Design review of the part shown in the three views and the two pictorial views. Dimensions are in mm from the part's minimum x, y and z. Round coordinates to 2 decimals unless told otherwise and drop trailing zeros. Loops run counter-clockwise (first coordinate to the right, second up) from the corner with the lowest first, then second, coordinate; pieces in that order, holes last. Notation, with made-up numbers: M -2,82 L 24,82 A7 cw 24,88 Z; hole C 18,86 d5. An arc over 180 degrees is marked long. One line per question, with ' | ' between items. Start each with the question number.
1) We need section C-C (z = 1.95). Give the boundary of the cut face in (x, y) (3 decimals).
2) We need section B-B (x = 50.8). Give the boundary of the cut face in (y, z) (3 decimals), and give its area (3 significant figures).
3) We need section D-D (y = 38.5). Give the boundary of the cut face in (x, z) (3 decimals), and give its area (3 significant figures).
4) For pin 1 Ø4 at (x, y) = (63.5, 38.1) entering from +Z; pin 2 Ø12 at (x, y) = (66.5, 6.5) entering from -Z, all flat-tipped, find the tip position at first contact; note any pin that passes through.
5) For probe 1 along X at (y, z) = (38.1, 2.15) (3 decimals); probe 2 along Y at (x, z) = (50.8, 0.9) (3 decimals); probe 3 along Y at (x, z) = (12.7, 1.2) (3 decimals), list the stretches that pass through material, from the lowest coordinate up. Write a range as from..to.
6) We need section A-A (y = 12.7). Give the boundary of the cut face in (x, z) (3 decimals).
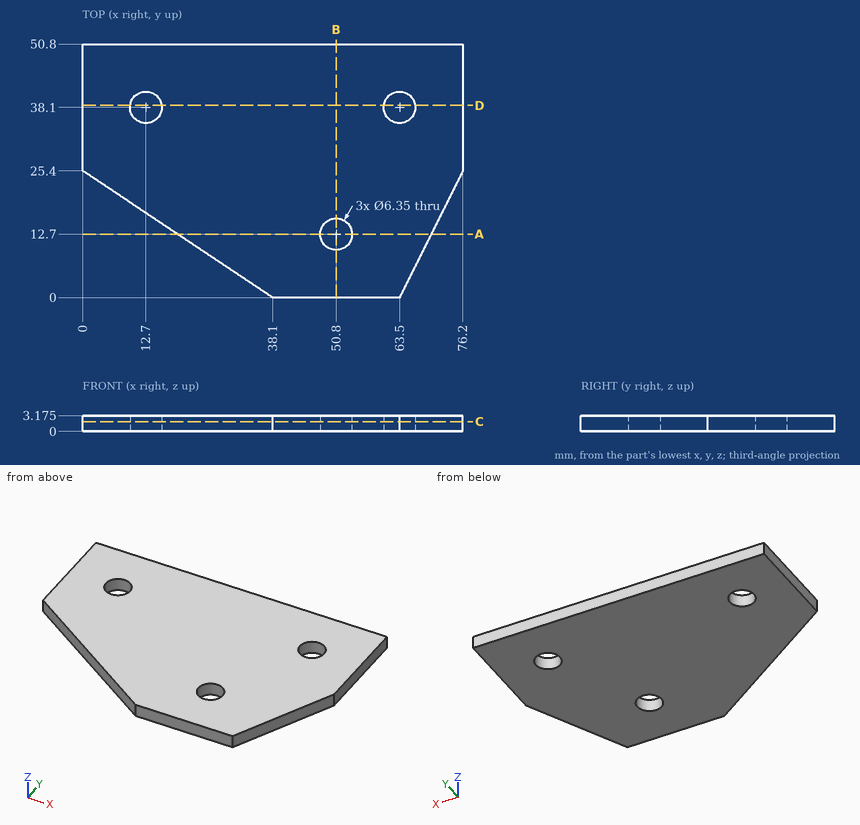
Answers below:
1) outline: M 0,25.4 L 38.1,0 L 63.5,0 L 76.2,25.4 L 76.2,50.8 L 0,50.8 Z; hole C 12.7,38.1 d6.35; hole C 50.8,12.7 d6.35; hole C 63.5,38.1 d6.35
2) outline: M 0,0 L 9.525,0 L 9.525,3.175 L 0,3.175 Z; M 15.875,0 L 50.8,0 L 50.8,3.175 L 15.875,3.175 Z | area: 141 mm^2
3) outline: M 0,0 L 9.55,0 L 9.55,3.175 L 0,3.175 Z; M 15.85,0 L 60.35,0 L 60.35,3.175 L 15.85,3.175 Z; M 66.65,0 L 76.2,0 L 76.2,3.175 L 66.65,3.175 Z | area: 202 mm^2
4) pin 1: through | pin 2: z = 0
5) probe 1: 0..9.525, 15.875..60.325, 66.675..76.2 | probe 2: 0..9.525, 15.875..50.8 | probe 3: 16.933..34.925, 41.275..50.8
6) outline: M 19.05,0 L 47.625,0 L 47.625,3.175 L 19.05,3.175 Z; M 53.975,0 L 69.85,0 L 69.85,3.175 L 53.975,3.175 Z
